CAD build for the part. Positions are in the model's coordinates, mm. A direction names the side the tool comes from. Round coordinates to 2 decimals unless told otherwise and drop trailing zeros. Order: outer loops, then holes, each group sorted by start corner. A loop starts at its lowest first (then second) coordinate and runs counter-clockwise, first axis right, second up. Notation, with made-up numbers: (49, -7.75) -> (56, -7.75) arc R33 ccw to (56, 27.25) -> close; hole circle Ø10 at (-39, -31). An arc over 180 degrees is marked (long way). Return JSON: item names as keys, results as strings. Group by question number.
Q1. Cut at B-B (x = -206). Write the cut outline in (y, z).
Q2. Which spindle directions (+Z, -Z, +X, -X, +Y, -Y) get a long thin tool onto all of the face, cutting with end or side? Do faces 1 (the flat face through (-98, -4, 95.6)), 2 (the flat face through (-99, -8.6, 99)), 3 (the flat face through (-99, -4, 98.85)), 4 (the flat face through (-139.436, -6, 5)), 5 (the flat face through (-126.6, -4, 98)). Say none if no direction does.
Q3. Cut at C-C (z = 80.1). Write the cut outline in (x, y), then the cut area to 3 significant figures.
Q4. Mould opens along X. For faces 6 (the flat face through (-120.2, -6, 6)), 7 (the flat face through (-55.6, -6, 8)), 8 (the flat face through (-113, -13.15, 6)) say: +X half, -X half, draft (parallel to the pull), parting line (faces both ways), or undercut.
Q5. Cut at D-D (x = -151). Write the cut outline in (y, z), then the cut area to 3 significant figures.
Q6. Cut at A-A (y = -6). Write the cut outline in (x, z), then the cut area to 3 significant figures.
Q7. Probe line 1 along X through (y, z) = (-7.75, 11.5); line 2 along X through (y, z) = (-12.25, 11); line 3 along X through (y, z) = (0.65, 102.1). List the from-to ranges inside material, lowest first.
Q8. Flat gauge pins, fed straight in: pin 1 (5 mm diameter, centred on x = -206, z = 4, fed in from -Y); pin 2 (3 mm diameter, centred on x = -114, y = -3, fed in from +Z); pin 3 (5.5 mm diameter, centred on y = -6, z = 8.5, fed in from -X). Where does each tip first touch, or does it go through?
Autodesk Inventor part; units mm, degrees
ref_plane "YZ Plane" through (0, 0, 0) normal (1, 0, 0) x (0, 1, 0)
ref_plane "XZ Plane" through (0, 0, 0) normal (0, 1, 0) x (-1, 0, 0)
ref_plane "XY Plane" through (0, 0, 0) normal (0, 0, 1) x (1, 0, 0)
sketch "Sketch1" plane through (0, 0, 0) normal (0, 1, 0) x (-1, 0, 0)
  line L0 (12, 105.1) -> (210, 105.1)
  line L1 (210, 105.1) -> (210, 0)
  line L2 (210, 0) -> (0, 0)
  circle A0 centre (4, 4) radius 1.5
  circle A1 centre (206, 4) radius 2
  circle A2 centre (206, 80.1) radius 2
  circle A3 centre (62.5, 102.1) radius 1.5
  line L3 (12, 105.1) -> (12, 100.9)
  line L4 (10, 98.9) -> (0, 98.9)
  arc A4 (10, 98.9) -> (12, 100.9) centre (10, 100.9) ccw
  line L5 (0, 98.9) -> (0, 0)
  point P0 (12, 98.9)
  dimension "d1" = 210
  dimension "d6" = 3
  dimension "d7" = 4
  dimension "d9" = 4
  dimension "d12" = 3
  dimension "d13" = 3
  dimension "d14" = 12
  dimension "d15" = 6.2
  dimension "d16" = 2
  dimension "d52" = 105.1
  dimension "d53" = 4
  dimension "d54" = 4
  dimension "d55" = 62.5
  dimension "d56" = 206
  dimension "d57" = 80.1
  dimension "d58" = 4
extrude "Extrusion1" add sketch "Sketch1" along normal blind 1.5
sketch "Sketch2" plane through (0, 0, 0) normal (0, -1, 0) x (1, 0, 0)
  line L0 (-126.6, 100.1) -> (-71, 100.1)
  line L1 (-71, 100.1) -> (-71, 95.6)
  line L2 (-71, 95.6) -> (-126.6, 95.6)
  line L3 (-126.6, 95.6) -> (-126.6, 100.1)
  line L4 (-210, 0) -> (-210, 105.1)
  line L5 (0, 98.9) -> (0, 0)
  line L6 (-72.8, 96.85) -> (-124.8, 96.85)
  line L7 (-124.8, 96.85) -> (-124.8, 98.85)
  line L8 (-124.8, 98.85) -> (-72.8, 98.85)
  line L9 (-72.8, 98.85) -> (-72.8, 96.85)
  line L10 (-210, 105.1) -> (-12, 105.1)
  point P0 (-126.6, 97.85)
  point P1 (-72.8, 97.85)
  point P2 (-71, 97.85)
  point P3 (-98.8, 98.85)
  point P4 (-98.8, 100.1)
  point P5 (-111, 105.1)
  dimension "d17" = 4.5
  dimension "d18" = 55.6
  dimension "d34" = 2
  dimension "d35" = 71
  dimension "d36" = 5
  dimension "d59" = 1.8
sketch "Sketch3" plane through (0, 0, 0) normal (0, -1, 0) x (1, 0, 0)
  line L0 (0, 0) -> (-210, 0)
  line L1 (-55.6, 0) -> (-86.6, 0)
  line L2 (-86.6, 0) -> (-86.6, 16)
  line L3 (-86.6, 16) -> (-55.6, 16)
  line L4 (-55.6, 16) -> (-55.6, 0)
  line L5 (0, 98.9) -> (0, 0)
  point P0 (-55.6, 8)
  point P1 (-86.6, 0)
  dimension "d23" = 55.6
  dimension "d24" = 31
  dimension "d25" = 16
extrude "Extrusion3" add sketch "Sketch3" along normal blind 12.5
sketch "Sketch4" plane through (0, 0, 0) normal (0, -1, 0) x (1, 0, 0)
  line L0 (-106.2, 0) -> (-120.2, 0)
  line L1 (-120.2, 0) -> (-120.2, 12.75)
  line L2 (-120.2, 12.75) -> (-106.2, 12.75)
  line L3 (-106.2, 12.75) -> (-106.2, 0)
  line L4 (-86.6, 16) -> (-86.6, 0)
  line L5 (0, 0) -> (-55.6, 0)
  line L6 (-86.6, 0) -> (-210, 0)
  dimension "d28" = 12.75
  dimension "d29" = 14
  dimension "d32" = 19.6
extrude "Extrusion4" add sketch "Sketch4" along normal blind 13.15
extrude "Extrusion5" add sketch "Sketch2" along normal blind 8.6
sketch "Sketch5" plane through (0, 0, 0) normal (0, -1, 0) x (1, 0, 0)
  line L0 (0, 0) -> (-210, 0)
  line L1 (-185, 0) -> (-173.5, 0)
  line L2 (-173.5, 0) -> (-173.5, 17)
  line L3 (-173.5, 17) -> (-185, 17)
  line L4 (-185, 17) -> (-185, 0)
  line L5 (-210, 0) -> (-210, 105.1)
  point P0 (-173.5, 0)
  dimension "d39" = 17
  dimension "d40" = 11.5
  dimension "d43" = 25
extrude "Extrusion6" add sketch "Sketch5" along normal blind 11
sketch "Sketch6" plane through (0, 0, 0) normal (0, -1, 0) x (1, 0, 0)
  line L0 (0, 0) -> (-210, 0)
  line L1 (-139.4357, 0) -> (-129.4357, 0)
  line L2 (-129.4357, 0) -> (-129.4357, 10)
  line L3 (-129.4357, 10) -> (-139.4357, 10)
  line L4 (-139.4357, 10) -> (-139.4357, 0)
  point P0 (-129.4357, 0)
  dimension "d44" = 10
  dimension "d45" = 10
extrude "Extrusion7" add sketch "Sketch6" along normal blind 12
sketch "Sketch7" plane through (0, 1.5, 0) normal (0, 0, -1) x (-1, 0, 0)
  circle A0 centre (134.4357, -7.5) radius 4.15
  line L0 (139.4357, -1.5) -> (139.4357, -13.5)
  line L1 (139.4357, -13.5) -> (129.4357, -13.5)
  point P0 (0, -1.5)
  point P1 (139.4357, -7.5)
  point P2 (134.4357, -13.5)
  dimension "d48" = 8.3
extrude "Extrusion8" add sketch "Sketch7" along normal blind 10
properties part number "motherboard"
Solution:
{
 "1": {"outline": "(0, 0) -> (1.5, 0) -> (1.5, 2) -> (0, 2) -> close; (0, 6) -> (1.5, 6) -> (1.5, 78.1) -> (0, 78.1) -> close; (0, 82.1) -> (1.5, 82.1) -> (1.5, 105.1) -> (0, 105.1) -> close"},
 "2": {"face 1": "+X, -X, -Y", "face 2": "+Z, +X, -X, -Y", "face 3": "-Y", "face 4": "+Z, -Z, -Y", "face 5": "+Z, -Z, -X, -Y"},
 "3": {"outline": "(-210, 0) -> (-208, 0) -> (-208, 1.5) -> (-210, 1.5) -> close; (-204, 0) -> (0, 0) -> (0, 1.5) -> (-204, 1.5) -> close", "area": "309 mm²"},
 "4": {"face 6": "undercut", "face 7": "+X half", "face 8": "draft"},
 "5": {"outline": "(0, 0) -> (1.5, 0) -> (1.5, 105.1) -> (0, 105.1) -> close", "area": "158 mm²"},
 "6": {"outline": "(-185, 0) -> (-173.5, 0) -> (-173.5, 17) -> (-185, 17) -> close; (-139.44, 0) -> (-138.59, 0) -> (-138.59, -10) -> (-130.29, -10) -> (-130.29, 0) -> (-129.44, 0) -> (-129.44, 10) -> (-139.44, 10) -> close; (-126.6, 95.6) -> (-71, 95.6) -> (-71, 100.1) -> (-126.6, 100.1) -> close; (-120.2, 0) -> (-106.2, 0) -> (-106.2, 12.75) -> (-120.2, 12.75) -> close; (-86.6, 0) -> (-55.6, 0) -> (-55.6, 16) -> (-86.6, 16) -> close; hole (-124.8, 96.85) -> (-72.8, 96.85) -> (-72.8, 98.85) -> (-124.8, 98.85) -> close", "area": "1,200 mm²"},
 "7": {"line 1": "x = -185 to -173.5, -120.2 to -106.2, -86.6 to -55.6", "line 2": "x = -120.2 to -106.2, -86.6 to -55.6", "line 3": "x = -210 to -64, -61 to -12"},
 "8": {"pin 1": "stops at y = 0", "pin 2": "stops at z = 100.1", "pin 3": "stops at x = -185"}
}
